Verification items for this drawing (mm, ordinates from the low corner). Round coordinates to 2 decimals unless told otherwise and drop trailing zeros. Loops run counter-clockwise (first coordinate to the right, second up) from the corner with the lowest first, then second, coordinate; pieces in that order, holes last. Notation, with made-up numbers: M -34,0 L 25,0 A22 ccw 25,19 Z; hole C 51.5,31.5 d7. An arc over 180 degrees is marked long. Answer as CSV lines item,"result".
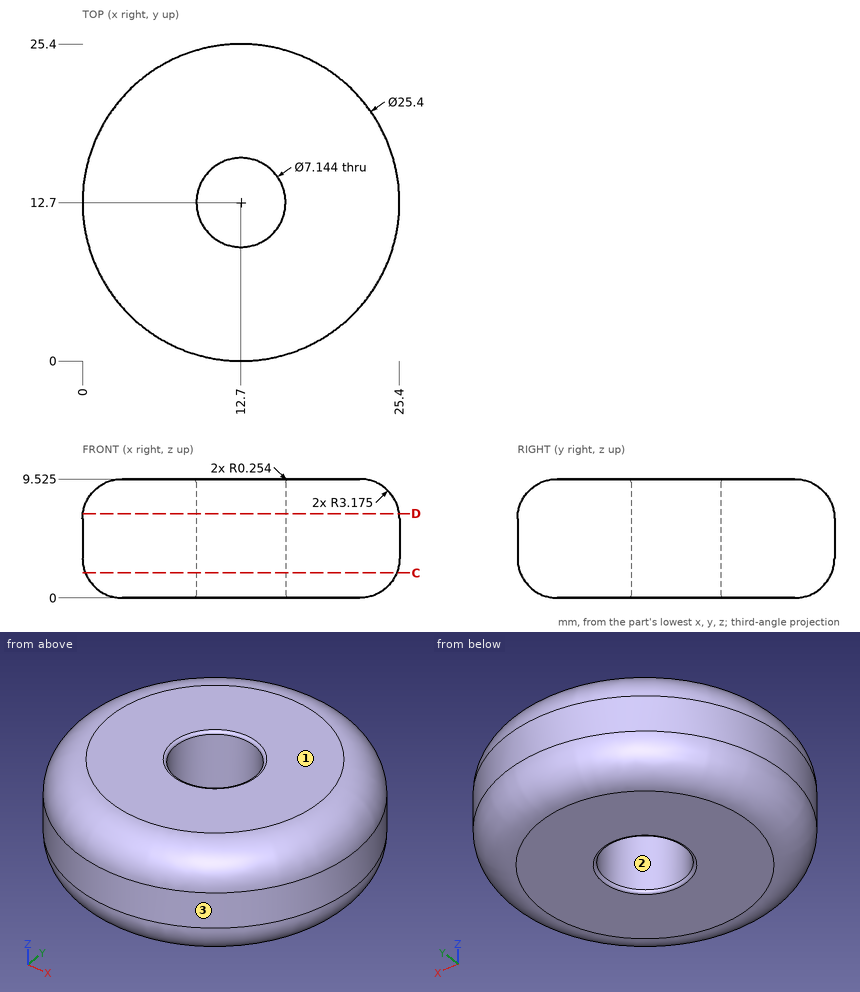
1) Draft check along Y on the marked faces 1, 2 and 3. Enter one of: +Y half, -Y half, draft (parallel to the pull), parting line (faces both ways), or undercut.
Here are the results:
face 1,"draft"
face 2,"undercut"
face 3,"parting line"
2) Material ranges on probe 1 along X at (y, z) = (12.7, 5); probe 2 along X at (y, z) = (14.25, 8.75), recorded low to high.
Here are the results:
probe 1,"x = 0 to 9.13, 16.27 to 25.4"
probe 2,"x = 1.2 to 9.48, 15.92 to 24.2"
3) Section check D-D (z = 6.75). Record the cut outline in (x, y) (1 decimal), plus the area to 3 significant figures.
Here are the results:
outline,"C 12.7,12.7 d25.3; hole C 12.7,12.7 d7.1"
area,"465 mm^2"
4) Go/stop test with flat-tipped pins: pin 1 (3 mm diameter, centred on x = 3.5, z = 2.5, fed in from -Y); pin 2 (1 mm diameter, centred on x = 11.5, z = 4.5, fed in from -Y); pin 3 (5 mm diameter, centred on y = 3, z = 1.5, fed in from -X). Record where each tip stops, or that it passes through.
Here are the results:
pin 1,"stops at y = 2.65"
pin 2,"stops at y = 0.02"
pin 3,"stops at x = 2.47"
5) Section check C-C (z = 2). Record the cut outline in (x, y) (1 decimal).
Here are the results:
outline,"C 12.7,12.7 d24.9; hole C 12.7,12.7 d7.1"
